Design review of the part shown in the three views and the two pictorial views. Dimensions are in mm from the part's minimum x, y and z. A direction names the side the tool comes from. Give positions to 0.01 mm unless a question says otherwise; leave off trailing zeros. Write each loop counter-clockwise with the first axis right and the second up, starting at its lowest first coordinate (ties: lowest second). Pieces come first, ordered by that corner, then holes. Notation, with made-up numbers: M -7,0.25 L 48,0.25 A12 ccw 48,9.25 Z; hole C -14,67.25 d1. An arc over 180 degrees is marked long. Use one line per item in the form item = value. Start each with the question number.
Q1. Clearance check with flat-ended pins moving along their axes: pin 1 Ø2 at (x, y) = (1.5, 10) entering from +Z; pin 2 Ø2 at (x, y) = (2, 2) entering from -Z; pin 3 Ø1.7 at (x, z) = (3, 4) entering from -Y. State where each tip first meets the part, or that it passes through.
Q2. Consider section A-A on y = 10.75. Write out the cut boundary in (x, z).
Q3. Mouldability with a two-part tool opening along Y and no side actions: class the marked faces 1, 2 and 3 as released by +Y, released by -Y, zero draft, split by the parting line, or undercut.
Q4. Tool access review of the marked faces 4 and 5: name each direction out of +Z, -Z, +X, -X, +Y, -Y from which nothing blocks a thin tool from reaching the whole face with its end or side.
Q5. For probe 1 along Y at (x, z) = (1, 3.75); probe 2 along X at (y, z) = (6.5, 3); probe 3 along Z at (x, y) = (3.5, 9.5), list the stretches that pass through material, from the lowest coordinate up. Write a range as [from, to].
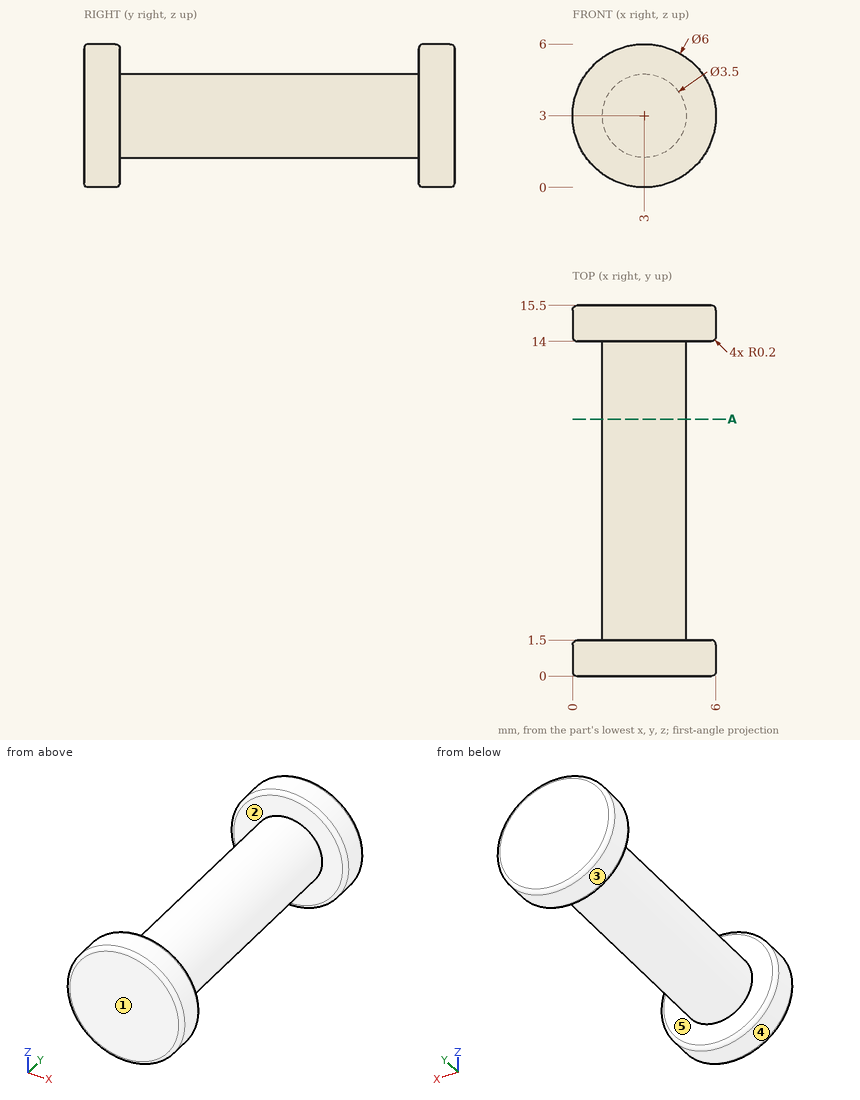
Working result:
q1.pin_1 = 4.68
q1.pin_2 = 0.01
q1.pin_3 = 0
q2.outline = C 3,3 d3.5
q3.face_1 = released by -Y
q3.face_2 = undercut
q3.face_3 = zero draft
q4.face_4 = +Y, -Y
q4.face_5 = none
q5.probe_1 = [0, 1.5], [14, 15.5]
q5.probe_2 = [1.25, 4.75]
q5.probe_3 = [1.32, 4.68]
